```python
from build123d import *

# Parameters (mm, degrees)
F1_DEPTH = 12.7
F2_DEPTH = 50.8
F3_W     = 25.4
F3_H     = 63.538220574
F3_R     = 6.858
F4_DEPTH = 12.7


with BuildPart() as f1:
    # F0 (on Front) → F1 (new body)
    with BuildSketch(Plane.XZ):
        with BuildLine():
            ThreePointArc((-37.4815943599, 31.75), (-69.2315943599, 0), (-37.4815943599, -31.75))
            Line((-37.4815943599, -31.75), (-37.4815943599, -12.7))
            ThreePointArc((-37.4815943599, -12.7), (-50.1815943599, 0), (-37.4815943599, 12.7))
            Line((-37.4815943599, 12.7), (-37.4815943599, 31.75))
        make_face()
        with BuildLine():
            Line((-37.4815943599, -12.7), (-37.4815943599, -31.75))
            ThreePointArc((-37.4815943599, -31.75), (-15.0309540572, -22.4506403027), (-5.7315943599, 0))
            ThreePointArc((-5.7315943599, 0), (-15.0309540572, 22.4506403027), (-37.4815943599, 31.75))
            Line((-37.4815943599, 31.75), (-37.4815943599, 12.7))
            ThreePointArc((-37.4815943599, 12.7), (-28.5013382388, 8.9802561211), (-24.7815943599, 0))
            ThreePointArc((-24.7815943599, 0), (-28.5013382388, -8.9802561211), (-37.4815943599, -12.7))
        make_face()
        with BuildLine():
            Line((-37.4815943599, -31.75), (-37.4815943599, -31.7906037465))
            Line((-37.4815943599, -31.7906037465), (37.4815943599, -31.7906037465))
            Line((37.4815943599, -31.7906037465), (37.4815943599, 31.7906037465))
            Line((37.4815943599, 31.7906037465), (-37.4815943599, 31.7906037465))
            Line((-37.4815943599, 31.7906037465), (-37.4815943599, 31.75))
            ThreePointArc((-37.4815943599, 31.75), (-15.0309540572, 22.4506403027), (-5.7315943599, 0))
            ThreePointArc((-5.7315943599, 0), (-15.0309540572, -22.4506403027), (-37.4815943599, -31.75))
        make_face()
    extrude(amount=F1_DEPTH)

    # F0 (on Front) → F2 (join)
    with BuildSketch(Plane.XZ):
        with BuildLine():
            Line((-37.4815943599, -12.7), (-37.4815943599, -31.75))
            ThreePointArc((-37.4815943599, -31.75), (-15.0309540572, -22.4506403027), (-5.7315943599, 0))
            ThreePointArc((-5.7315943599, 0), (-15.0309540572, 22.4506403027), (-37.4815943599, 31.75))
            Line((-37.4815943599, 31.75), (-37.4815943599, 12.7))
            ThreePointArc((-37.4815943599, 12.7), (-28.5013382388, 8.9802561211), (-24.7815943599, 0))
            ThreePointArc((-24.7815943599, 0), (-28.5013382388, -8.9802561211), (-37.4815943599, -12.7))
        make_face()
        with BuildLine():
            ThreePointArc((-37.4815943599, 31.75), (-69.2315943599, 0), (-37.4815943599, -31.75))
            Line((-37.4815943599, -31.75), (-37.4815943599, -12.7))
            ThreePointArc((-37.4815943599, -12.7), (-50.1815943599, 0), (-37.4815943599, 12.7))
            Line((-37.4815943599, 12.7), (-37.4815943599, 31.75))
        make_face()
    extrude(amount=-F2_DEPTH)

    # F3 (on face) → F4 (join)
    with BuildSketch(Plane.YZ.offset(37.4815943599)):
        with Locations((-25.4, 0.0214934595)):
            Rectangle(F3_W, F3_H)
        with Locations((-22.8328048199, -12.7)):
            Circle(F3_R, mode=Mode.SUBTRACT)
        with Locations((-22.8328048199, 12.7)):
            Circle(F3_R, mode=Mode.SUBTRACT)
    extrude(amount=-F4_DEPTH)


solid = f1.part
```
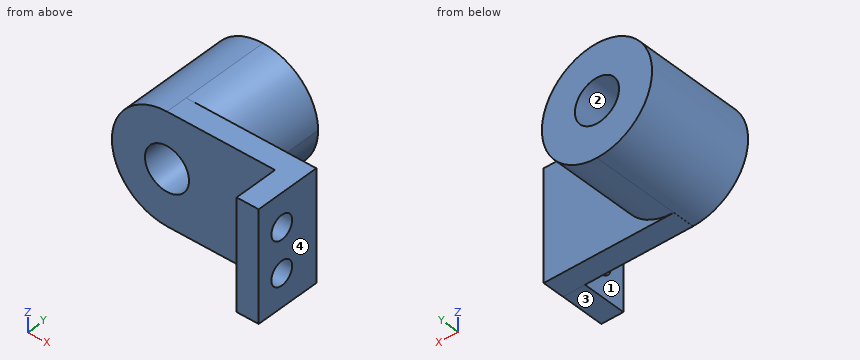
Here's how the part is built. I have some questions about the finished solid (model axes, mm). Face numbers are marked on the shaded views. Coordinates: 2 decimals unless noted, no trailing zeros. Order: outer loops, then holes, each group sorted by start corner. A loop starts at its lowest first (then second) coordinate and runs counter-clockwise, first axis right, second up.
1) Imagine slicing it at A-A on y = -2. List the corners of the cut face in (x, z) for me.
2) Imagine slicing it at D-D on z = -21. List the corners of the cut face in (x, y) for me, and give its area (3 significant figures).
3) We'd pull the mould along X, two halves only. Please class the marked faces 1, 2, 3 and 4: +X half, -X half, draft (parallel to the pull), parting line (faces both ways), or undercut.
4) Will these pins go through, and if not, where does the flat tip stop? pin 1 (14 mm diameter, centred on x = 32, y = -25, fed in from -Z); pin 2 (2 mm diameter, centred on x = 4, z = -1.5, fed in from -Y); pin 3 (1.5 mm diameter, centred on x = 23, z = -10.5, fed in from +Y); pin 4 (23 mm diameter, centred on x = -37.48, z = 0, fed in from +Y).
5) I need wall thicknesses on line 1 (Z direction, x = 25.5, y = -20); line 2 (X direction, y = -16.5, z = -20.5); line 3 (Y direction, x = -60.5, z = 11.5). Which ranges of each line are inside material? Lowest first, please.
6) Imagine slicing it at C-C on x = 20. List the corners of the cut face in (y, z) for me.
Response values:
1. outline: (-37.48, -31.79) - (37.48, -31.79) - (37.48, 31.79) - (-37.48, 31.79) - (-37.48, 31.75) arc R31.75 ccw to (-37.48, -31.75) - close; hole circle Ø25.4 at (-37.48, 0)
2. outline: (-61.29, -12.7) - (24.78, -12.7) - (24.78, -38.1) - (37.48, -38.1) - (37.48, 0) - (-13.67, 0) - (-13.67, 50.8) - (-61.29, 50.8) - close
2. area: 4,000 mm2
3. face 1: -X half
3. face 2: undercut
3. face 3: draft
3. face 4: +X half
4. pin 1: stops at z = -31.75
4. pin 2: stops at y = -12.7
4. pin 3: stops at y = 0
4. pin 4: passes through
5. line 1: z = -31.75 to -18.95, -6.45 to 6.45, 18.95 to 31.79
5. line 2: x = 24.78 to 37.48
5. line 3: y = -12.7 to 50.8
6. outline: (-12.7, -31.79) - (0, -31.79) - (0, 31.79) - (-12.7, 31.79) - close
